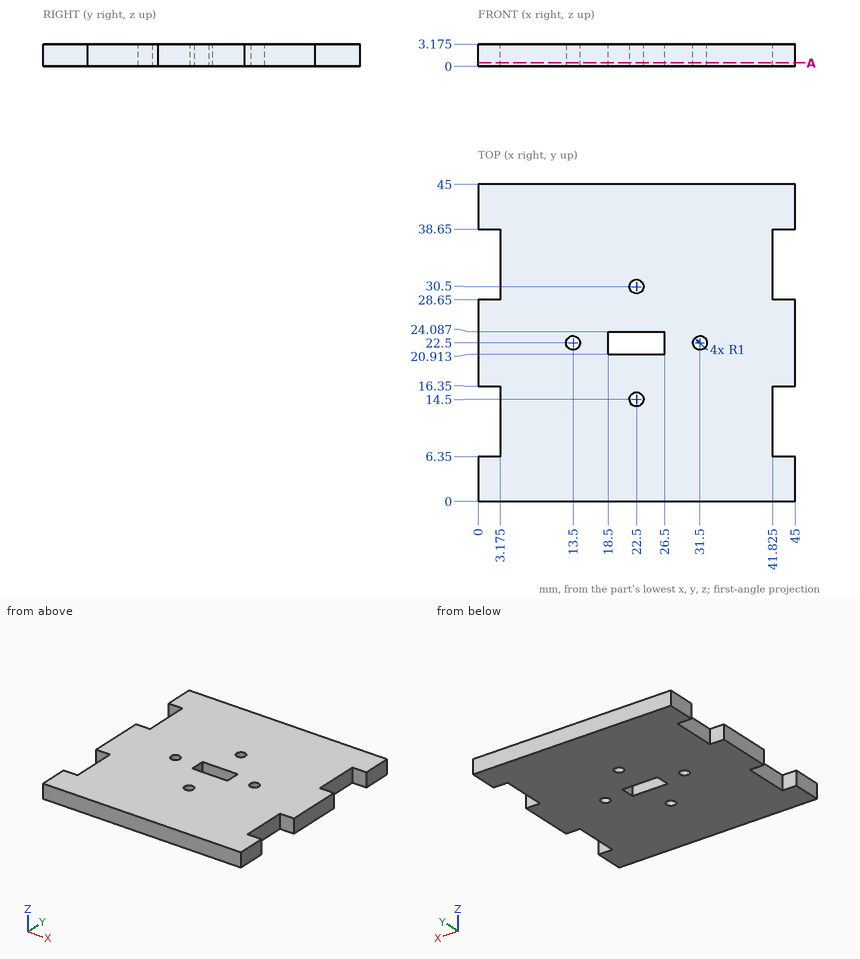
For this review, use the dimensioned drawing (mm, ordinates from the lowest corner) and the shaded views. Round coordinates to 2 decimals unless told otherwise and drop trailing zeros. Use CSV: the item, a comma, the result in double quotes.
(1) To check wall thickness, follow L1, parallel to Y at x = 42.5, z = 1.75; L2, parallel to X at y = 22, z = 2.3 (1 decimal); L3, parallel to Y at x = 20, z = 1.05. State the ranges of each line that lie inside material, in increasing order. Write a range as [from, to].
Computed values:
L1,"[0, 6.35], [16.35, 28.65], [38.65, 45]"
L2,"[0, 12.6], [14.4, 18.5], [26.5, 30.6], [32.4, 45]"
L3,"[0, 20.91], [24.09, 45]"
(2) Clearance check with flat-ended pins moving along their axes: P1, Ø1.6, axis at x = 1.5, z = 1.5, coming from the -Y side; P2, Ø1, axis at y = 32, z = 1.5, coming from the -X side (1 decimal); P3, Ø1, axis at y = 7, z = 2.5, coming from the +X side (1 decimal). State where each tip first meets the part, or that it passes through.
Computed values:
P1,"y = 0"
P2,"x = 3.2"
P3,"x = 41.8"
(3) Consider section A-A, the plane z = 0.5. Give the number of separate pieces and of enclosed holes in the cut face, plus the area to 3 significant figures.
Computed values:
separate pieces,"1"
enclosed holes,"5"
area,"1,860 mm²"
